from build123d import *

# Parameters (mm, degrees)
F1_DEPTH = 60


with BuildPart() as f1:
    # F0 (on Front) → F1 (new body, symmetric)
    with BuildSketch(Plane.XZ):
        with BuildLine():
            Line((49.355, 12.725), (51.5, 12.725))
            Line((51.5, 12.725), (51.5, 23.5))
            ThreePointArc((51.5, 23.5), (50.62132, 25.62132), (48.5, 26.5))
            Line((48.5, 26.5), (-48.5, 26.5))
            ThreePointArc((-48.5, 26.5), (-50.62132, 25.62132), (-51.5, 23.5))
            Line((-51.5, 23.5), (-51.5, 12.725))
            Line((-51.5, 12.725), (-49.355, 12.725))
            Line((-49.355, 12.725), (-49.355, 14.725))
            Line((-49.355, 14.725), (-45.5, 14.725))
            Line((-45.5, 14.725), (-45.5, 16.725))
            Line((-45.5, 16.725), (-49.355, 16.725))
            Line((-49.355, 16.725), (-49.355, 18.725))
            Line((-49.355, 18.725), (-45.5, 18.725))
            Line((-45.5, 18.725), (-45.5, 24.21))
            Line((-45.5, 24.21), (45.5, 24.21))
            Line((45.5, 24.21), (45.5, 18.725))
            Line((45.5, 18.725), (49.355, 18.725))
            Line((49.355, 18.725), (49.355, 16.725))
            Line((49.355, 16.725), (45.5, 16.725))
            Line((45.5, 16.725), (45.5, 14.725))
            Line((45.5, 14.725), (49.355, 14.725))
            Line((49.355, 14.725), (49.355, 12.725))
        make_face()
        Polygon((-51.5, 12.725), (-51.5, -12.725), (-49.355, -12.725), (-36.5, -12.725), (-36.5, 12.725), (-49.355, 12.725), align=None)
        with BuildLine():
            Line((-48.5, -26.5), (48.5, -26.5))
            ThreePointArc((48.5, -26.5), (50.62132, -25.62132), (51.5, -23.5))
            Line((51.5, -23.5), (51.5, -12.725))
            Line((51.5, -12.725), (49.355, -12.725))
            Line((49.355, -12.725), (49.355, -14.725))
            Line((49.355, -14.725), (45.5, -14.725))
            Line((45.5, -14.725), (45.5, -16.725))
            Line((45.5, -16.725), (49.355, -16.725))
            Line((49.355, -16.725), (49.355, -18.725))
            Line((49.355, -18.725), (45.5, -18.725))
            Line((45.5, -18.725), (45.5, -24.21))
            Line((45.5, -24.21), (-45.5, -24.21))
            Line((-45.5, -24.21), (-45.5, -18.725))
            Line((-45.5, -18.725), (-49.355, -18.725))
            Line((-49.355, -18.725), (-49.355, -16.725))
            Line((-49.355, -16.725), (-45.5, -16.725))
            Line((-45.5, -16.725), (-45.5, -14.725))
            Line((-45.5, -14.725), (-49.355, -14.725))
            Line((-49.355, -14.725), (-49.355, -12.725))
            Line((-49.355, -12.725), (-51.5, -12.725))
            Line((-51.5, -12.725), (-51.5, -23.5))
            ThreePointArc((-51.5, -23.5), (-50.62132, -25.62132), (-48.5, -26.5))
        make_face()
        Polygon((49.355, -12.725), (51.5, -12.725), (51.5, 12.725), (49.355, 12.725), (36.5, 12.725), (36.5, -12.725), align=None)
    extrude(amount=F1_DEPTH, both=True)


solid = f1.part
Input: part model. Units: mm. Frame: model coordinates. A direction names the side the tool comes from. Give positions to 0.01 mm unless a question says otherwise; leave off trailing zeros. Write each loop counter-clockwise with the first axis right and the second up, starting at its lowest first coordinate (ties: lowest second). Pieces come first, ordered by that corner, then holes.
Q1. Section A-A, the plane z = 0.5. Output: boundary loops of the cut face in (x, y).
Q2. Section B-B, the plane x = -40.5. Output: boundary loops of the cut face in (y, z) (3 decimals), plus the area to 3 significant figures.
Q3. Set-up query: faces 1 (the face through (-1, -1, 24.21)), 2 (the face through (0, 60, 26)). Return all of +Z, -Z, +X, -X, +Y, -Y with unobstructed straight access to the full face (end or side cutting, diameter ignored); none if empty.
Q4. Pull-direction query (Z, two-part tool) for faces 3 (the face through (-1, -1, -26.5)), 4 (the face through (-45.5, -1, 21)), 5 (the face through (0, -60, 26)); classes: pulls with the +Z half, pulls with the -Z half, needs draft (parallel to the pull), parting line crosses it, or undercut.
Q5. Material intervals for probe 1 along Z at (x, y) = (-44, -3) (3 decimals); probe 2 along X at (y, z) = (50.5, -6); probe 3 along X at (y, z) = (22.5, 18) (3 decimals), sorted ascending.
Q6. Section C-C, the plane x = -18. Output: boundary loops of the cut face in (y, z).
Filled in:
1. outline: (-51.5, -60) - (-36.5, -60) - (-36.5, 60) - (-51.5, 60) - close; (36.5, -60) - (51.5, -60) - (51.5, 60) - (36.5, 60) - close
2. outline: (-60, -26.5) - (60, -26.5) - (60, -24.21) - (-60, -24.21) - close; (-60, -12.725) - (60, -12.725) - (60, 12.725) - (-60, 12.725) - close; (-60, 24.21) - (60, 24.21) - (60, 26.5) - (-60, 26.5) - close
2. area: 3,600 mm2
3. face 1: +Y, -Y
3. face 2: +Z, -Z, +X, -X, +Y
4. face 3: pulls with the -Z half
4. face 4: undercut
4. face 5: needs draft
5. probe 1: z = -26.5 to -24.21, -12.725 to 12.725, 24.21 to 26.5
5. probe 2: x = -51.5 to -36.5, 36.5 to 51.5
5. probe 3: x = -51.5 to -49.355, 49.355 to 51.5
6. outline: (-60, -26.5) - (60, -26.5) - (60, -24.21) - (-60, -24.21) - close; (-60, 24.21) - (60, 24.21) - (60, 26.5) - (-60, 26.5) - close
